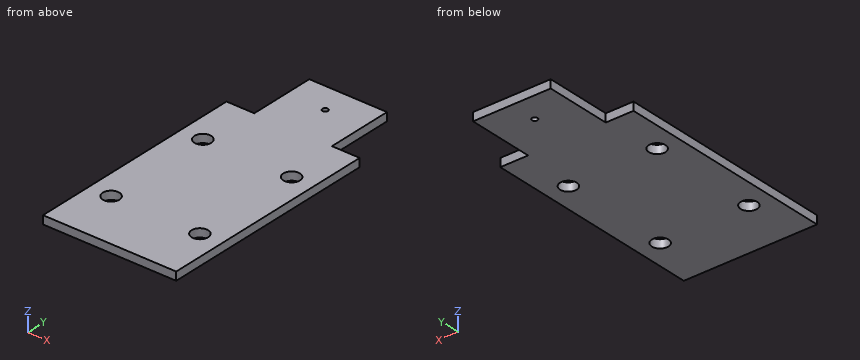
from build123d import *

# Parameters (mm, degrees)
F0_W     = 152.4
F0_H     = 254
F0_R     = 9.525
F1_DEPTH = 9.525
F2_W     = 88.9
F2_H     = 9.525
F3_DEPTH = 76.2
F4_R     = 3.175
F5_DEPTH = 9.526


with BuildPart() as f1:
    # F0 (on Top) → F1 (new body)
    with BuildSketch(Plane.XY):
        Rectangle(F0_W, F0_H)
        with Locations((-50.8, -63.5)):
            Circle(F0_R, mode=Mode.SUBTRACT)
        with Locations((50.8, -63.5)):
            Circle(F0_R, mode=Mode.SUBTRACT)
        with Locations((-50.8, 63.5)):
            Circle(F0_R, mode=Mode.SUBTRACT)
        with Locations((50.8, 63.5)):
            Circle(F0_R, mode=Mode.SUBTRACT)
    extrude(amount=F1_DEPTH)

    # F2 (on face) → F3 (join)
    with BuildSketch(Plane(origin=(0, 127, 0), x_dir=(-1, 0, 0), z_dir=(0, 1, 0))):
        with Locations((0, 4.7625)):
            Rectangle(F2_W, F2_H)
    extrude(amount=F3_DEPTH)

    # F4 (on face) → F5 (cut, through all)
    with BuildSketch(Plane.XY.offset(9.525)):
        with Locations((0, 171.45)):
            Circle(F4_R)
    extrude(amount=-F5_DEPTH, mode=Mode.SUBTRACT)


solid = f1.part
Verification items for the finished model (mm, model axes). Give positions to 0.01 mm unless a question says otherwise; leave off trailing zeros. Loops run counter-clockwise (first coordinate to the right, second up) from the corner with the lowest first, then second, coordinate; pieces in that order, holes last. Notation, with made-up numbers: (-31, 59) - (-27, 59) arc R29 cw to (-27, 95) - close; hole circle Ø3 at (-17, 3.25). An arc over 180 degrees is marked (long way). Write each question's results on one line, items separated by ' | '.
1) Depth check by flat-ended pin: P1, Ø15, axis at x = 50.8, y = -63.5, coming from the +Z side; P2, Ø3, axis at y = 166, z = 4.5, coming from the +X side. Enter the tip coordinate at first touch or a pass-through.
Solution:
P1: through | P2: x = 44.45
2) Material ranges on L1, parallel to Y at x = -50.8, z = 2.25 (3 decimals); L2, parallel to X at y = 171.45, z = 2 (3 decimals); L3, parallel to X at y = -70, z = 0.75, recorded low to high. Write a range as from..to.
Solution:
L1: -127..-73.025, -53.975..53.975, 73.025..127 | L2: -44.45..-3.175, 3.175..44.45 | L3: -76.2..-57.76, -43.84..43.84, 57.76..76.2
3) Sectioned sample at C-C on y = 63.5. Record the boundary of the cut face in (x, z) (3 decimals), plus the area to 3 significant figures.
Solution:
outline: (-76.2, 0) - (-60.325, 0) - (-60.325, 9.525) - (-76.2, 9.525) - close; (-41.275, 0) - (41.275, 0) - (41.275, 9.525) - (-41.275, 9.525) - close; (60.325, 0) - (76.2, 0) - (76.2, 9.525) - (60.325, 9.525) - close | area: 1,090 mm2
4) Sectioned sample at D-D on z = 6. Record the boundary of the cut face in (x, y) (3 decimals).
Solution:
outline: (-76.2, -127) - (76.2, -127) - (76.2, 127) - (44.45, 127) - (44.45, 203.2) - (-44.45, 203.2) - (-44.45, 127) - (-76.2, 127) - close; hole circle Ø19.05 at (-50.8, -63.5); hole circle Ø19.05 at (-50.8, 63.5); hole circle Ø6.35 at (0, 171.45); hole circle Ø19.05 at (50.8, -63.5); hole circle Ø19.05 at (50.8, 63.5)
5) Sectioned sample at A-A on x = -50.8. Record the boundary of the cut face in (y, z) (3 decimals), plus the area to 3 significant figures.
Solution:
outline: (-127, 0) - (-73.025, 0) - (-73.025, 9.525) - (-127, 9.525) - close; (-53.975, 0) - (53.975, 0) - (53.975, 9.525) - (-53.975, 9.525) - close; (73.025, 0) - (127, 0) - (127, 9.525) - (73.025, 9.525) - close | area: 2,060 mm2
6) Sectioned sample at B-B on x = 0. Record the boundary of the cut face in (y, z) (3 decimals), plus the area to 3 significant figures.
Solution:
outline: (-127, 0) - (168.275, 0) - (168.275, 9.525) - (-127, 9.525) - close; (174.625, 0) - (203.2, 0) - (203.2, 9.525) - (174.625, 9.525) - close | area: 3,080 mm2
